from build123d import *

# Parameters (mm, degrees)
SKETCH1_W           = 3.1
SKETCH1_H           = 2
BOSS_EXTRUDE1_DEPTH = 4
CIRPATTERN1_COUNT   = 5


with BuildPart() as part:
    # Sketch1 → Revolve1 (revolve)
    with BuildSketch(Plane.XY, mode=Mode.PRIVATE) as revolve1_sk:
        Polygon((0, 35), (0, -35), (-4.9, -35), (-4.9, 31), (-12, 31), (-12, 35), align=None)
        with Locations((-6.45, -28.5)):
            Rectangle(SKETCH1_W, SKETCH1_H)
    revolve(revolve1_sk.sketch.rotate(Axis((0, -35, 0), (0, 1, 0)), 270), axis=Axis((0, -35, 0), (0, 1, 0)))

    # Sketch2 → Boss-Extrude1 (add)
    with BuildSketch(Plane(origin=(0, 35, 0), x_dir=(1, 0, 0), z_dir=(0, 1, 0))):
        with BuildLine():
            Line((-1.25, 11.934718262), (-1.25, 21.934718262))
            Line((-1.25, 21.934718262), (1.25, 21.934718262))
            Line((1.25, 21.934718262), (1.25, 11.934718262))
            ThreePointArc((1.25, 11.934718262), (0, 12), (-1.25, 11.934718262))
        make_face()
    boss_extrude1 = extrude(amount=-BOSS_EXTRUDE1_DEPTH)

    # CirPattern1: Boss-Extrude1 ×5 about axis
    cirpattern1_axis = Axis((0, 0, 0), (0, 1, 0))
    for i in range(1, CIRPATTERN1_COUNT):
        add(boss_extrude1.rotate(cirpattern1_axis, i * 360 / CIRPATTERN1_COUNT))


solid = part.part
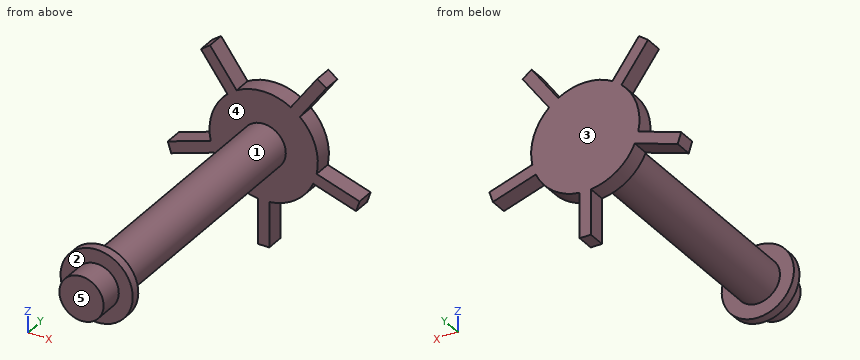
Source: CAD feature listing. Evaluate the final solid. Frame: model axes, mm. Face numbers are marked on the shaded views. A direction names the side the tool comes from. Round coordinates to 2 decimals unless told otherwise and drop trailing zeros. Loops run counter-clockwise (first coordinate to the right, second up) from the corner with the lowest first, then second, coordinate; pieces in that order, holes last. Notation, with made-up numbers: (-31, -17) - (-11, -17) arc R16 ccw to (-11, 8) - close; hole circle Ø4 at (-33, 39). An arc over 180 degrees is marked (long way). Write item = value, one per line. Start each with the question number.
Item 1: Section query A-A on x = -9. Output: boundary loops of the cut face in (y, z).
Item 2: Material intervals for line 1 (Y direction, x = 8, z = 3.5); line 2 (X direction, y = 32, z = -18); line 3 (X direction, y = -18, z = -4), sorted ascending.
Item 3: Mould query, pull axis Y, two halves, no side actions, for the marked faces 3, 4 and 5. Classes: released by +Y, released by -Y, zero draft, split by the parting line, or undercut.
Item 4: Section query C-C on x = 0. Output: boundary loops of the cut face in (y, z).
Item 5: Reachability of the marked faces 1 and 2 from +Z, -Z, +X, -X, +Y, -Y: full face, straight path, thin tool, end or side. Return the list, or none.
Item 6: Section query D-D on y = -25. Output: boundary loops of the cut face in (x, z).
Item 7: Section query B-B on z = 0. Output: boundary loops of the cut face in (x, y).
Item 8: First-contact query: pin 1 Ø1 at (x, y) = (-2, -21.5) entering from +Z; pin 2 Ø1.2 at (y, z) = (33, -16) entering from -X; pin 3 Ø1.5 at (y, z) = (-1, -4.5) entering from +X. Flat tips, straight axial feed; report the tip coordinate or a pass-through.
Results list:
q1.outline = (31, -7.94) - (35, -7.94) - (35, 7.94) - (31, 7.94) - close; (31, 10.26) - (35, 10.26) - (35, 14.51) - (31, 14.51) - close
q2.line_1 = 31 to 35
q2.line_2 = -1.25 to 1.25
q2.line_3 = -2.83 to 2.83
q3.face_3 = released by +Y
q3.face_4 = undercut
q3.face_5 = released by -Y
q4.outline = (-35, -4.9) - (-29.5, -4.9) - (-29.5, -8) - (-27.5, -8) - (-27.5, -4.9) - (31, -4.9) - (31, -21.93) - (35, -21.93) - (35, 12) - (31, 12) - (31, 4.9) - (-27.5, 4.9) - (-27.5, 8) - (-29.5, 8) - (-29.5, 4.9) - (-35, 4.9) - close
q5.face_1 = none
q5.face_2 = -Y
q6.outline = circle Ø9.8 at (0, 0)
q7.outline = (-12, 31) - (-4.9, 31) - (-4.9, -27.5) - (-8, -27.5) - (-8, -29.5) - (-4.9, -29.5) - (-4.9, -35) - (4.9, -35) - (4.9, -29.5) - (8, -29.5) - (8, -27.5) - (4.9, -27.5) - (4.9, 31) - (12, 31) - (12, 35) - (-12, 35) - close
q8.pin_1 = 4.66
q8.pin_2 = -1.25
q8.pin_3 = 3.15
